from build123d import *

# Parameters (mm, degrees)
SKETCH_2_R          = 30
EXTRUDE_1_DEPTH     = 4
SKETCH_3_R          = 3.5
CUT_EXTRUDE_1_DEPTH = 4
SKETCH_14_W         = 20.5
SKETCH_14_H         = 2.5
EXTRUDE_2_DEPTH     = 80
SKETCH_15_W         = 20.5
SKETCH_15_H         = 2.5
EXTRUDE_3_DEPTH     = 20
FILLET_1_R          = 5
FILLET_3_R          = 1


with BuildPart() as part:
    # 草图2 → 凸台-拉伸1 (new body)
    with BuildSketch(Plane.XY):
        Circle(SKETCH_2_R)
    extrude(amount=EXTRUDE_1_DEPTH)

    # 草图3 → 切除-拉伸1 (cut)
    with BuildSketch(Plane.XY.offset(4)):
        with Locations((-17.67766953, 17.67766953)):
            Circle(SKETCH_3_R)
        with Locations(Location((17.67766953, 17.67766953, 0), (0, 0, 180))):
            Circle(SKETCH_3_R)
        with Locations((17.67766953, -17.67766953)):
            Circle(SKETCH_3_R)
        with Locations(Location((-17.67766953, -17.67766953, 0), (0, 0, 180))):
            Circle(SKETCH_3_R)
    extrude(amount=-CUT_EXTRUDE_1_DEPTH, mode=Mode.SUBTRACT)

    # 草图14 → 凸台-拉伸2 (add)
    with BuildSketch(Plane.XY):
        Rectangle(SKETCH_14_W, SKETCH_14_H)
    extrude(amount=EXTRUDE_2_DEPTH)

    # 草图15 → 凸台-拉伸3 (add)
    with BuildSketch(Plane(origin=(0, 0, 0), x_dir=(1, 0, 0), z_dir=(0, 1, 0))):
        with Locations((0, -78.75)):
            Rectangle(SKETCH_15_W, SKETCH_15_H)
    extrude(amount=EXTRUDE_3_DEPTH)

    # 圆角1
    fillet_1_edges = [part.edges().sort_by_distance(p)[0] for p in [
        (0, 1.25, 4),
        (0, -1.25, 4),
        (0, 1.25, 77.5),
    ]]
    fillet(fillet_1_edges, radius=FILLET_1_R)

    # 圆角3
    fillet_3_edges = [part.edges().sort_by_distance(p)[0] for p in [
        (0, -1.25, 80),
        (0, 20, 80),
        (0, 20, 77.5),
    ]]
    fillet(fillet_3_edges, radius=FILLET_3_R)


solid = part.part
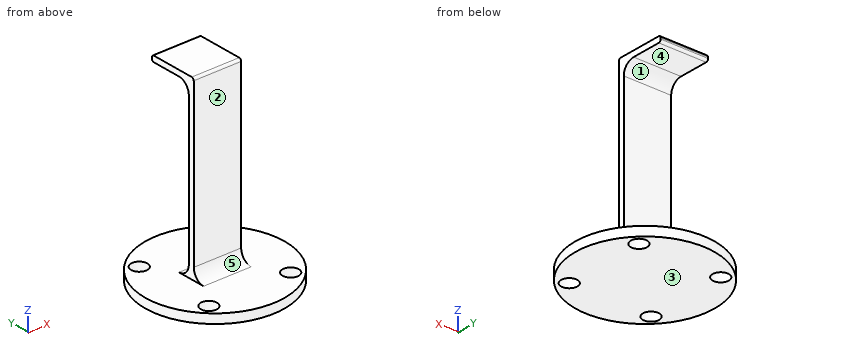
Could you check a few things on this model? Use its own coordinates, in mm. Face numbers are marked on the shaded views. A direction names the side the tool comes from. Round coordinates to 2 decimals unless told otherwise and drop trailing zeros. Write each loop counter-clockwise with the first axis right and the second up, starting at its lowest first coordinate (ties: lowest second). Pieces come first, ordered by that corner, then holes. Notation, with made-up numbers: (53.5, 24) - (70.5, 24) arc R23 ccw to (70.5, 43) - close; hole circle Ø7 at (72, -28.5). An arc over 180 degrees is marked (long way). Use a Markdown table: item, result.
Q1. For pin 1 (12 mm diameter, centred on x = 20.5, y = -14, fed in from +Z); pin 2 (6 mm diameter, centred on x = 3.5, z = 32, fed in from -Y); pin 3 (6 mm diameter, centred on x = -1, z = 40.5, fed in from +Y), each with a flat end and sliding along its axis, tell me the tip position at first contact or that it passes through.
Output values:
| item | result |
|---|---|
| pin 1 | z = 4 |
| pin 2 | y = -1.25 |
| pin 3 | y = 1.25 |
Q2. I want a section at B-B (x = 0). List the corners of the cut face in (y, z) for me, plus the area to 3 significant figures.
Output values:
| item | result |
|---|---|
| outline | (-30, 0) - (30, 0) - (30, 4) - (6.25, 4) arc R5 cw to (1.25, 9) - (1.25, 72.5) arc R5 cw to (6.25, 77.5) - (19, 77.5) arc R1 ccw to (20, 78.5) - (20, 79) arc R1 ccw to (19, 80) - (-0.25, 80) arc R1 ccw to (-1.25, 79) - (-1.25, 9) arc R5 cw to (-6.25, 4) - (-30, 4) - close |
| area | 492 mm2 |
Q3. For the marked faces 4 and 5, which set-ups out of +Z, -Z, +X, -X, +Y, -Y let a thin tool reach every point of the face, with its end or its side?
Output values:
| item | result |
|---|---|
| face 4 | +X, -X, +Y |
| face 5 | +Z, +X, -X, -Y |
Q4. Thinking about a two-plate mould opening in Z: for the marked faces 1, 2 and 3, which applies, released by +Z, released by -Z, zero draft, split by the parting line, or undercut?
Output values:
| item | result |
|---|---|
| face 1 | undercut |
| face 2 | zero draft |
| face 3 | released by -Z |
Q5. I want a section at A-A (y = 7.5). List the corners of the cut face in (x, z) for me, plus the area to 3 significant figures.
Output values:
| item | result |
|---|---|
| outline | (-29.05, 0) - (29.05, 0) - (29.05, 4) - (-29.05, 4) - close; (-10.25, 77.5) - (10.25, 77.5) - (10.25, 80) - (-10.25, 80) - close |
| area | 284 mm2 |
Q6. Please list where these lines run through material, in increasing order: L1, parallel to Z at x = 7, y = -26.5; L2, parallel to Y at x = 1, z = 13.5; L3, parallel to Z at x = -3, y = 14.5.
Output values:
| item | result |
|---|---|
| L1 | 0 to 4 |
| L2 | -1.25 to 1.25 |
| L3 | 0 to 4, 77.5 to 80 |
Q7. I want a section at D-D (y = -13). List the corners of the cut face in (x, z) for me.
Output values:
| item | result |
|---|---|
| outline | (-27.04, 0) - (27.04, 0) - (27.04, 4) - (-27.04, 4) - close |
Q8. I want a section at C-C (z = 32). List the corners of the cut face in (x, y) for me.
Output values:
| item | result |
|---|---|
| outline | (-10.25, -1.25) - (10.25, -1.25) - (10.25, 1.25) - (-10.25, 1.25) - close |
